For this review, take the finished solid that the model builds, in its own axes (mm). Give positions to 0.01 mm unless a question says otherwise; leave off trailing zeros. Write each loop counter-clockwise with the first axis right and the second up, starting at its lowest first coordinate (ties: lowest second). Pieces come first, ordered by that corner, then holes.
1) We need section B-B on y = 77.5. Give the boundary of the cut face in (x, z).
2) We need section A-A on x = 127. Give the boundary of the cut face in (y, z), and give its area (3 significant figures).
3) We need section C-C on x = 61. Give the boundary of the cut face in (y, z), and give its area (3 significant figures).
4) Wall thickness on line 1 along X through (y, z) = (184.5, 2.3); line 2 along Y through (x, z) = (13, 2.35): over which ranges is each line inside the solid? List them lowest first.
5) We need section D-D on y = 158.5. Give the boundary of the cut face in (x, z), and give its area (3 significant figures).
6) For P1, Ø10, axis at x = 113, y = 106.5, coming from the -Z side; P2, Ø6, axis at x = 174.5, y = 181.5, coming from the +Z side; P3, Ø17, axis at x = 168, y = 105.5, coming from the +Z side, all flat-tipped, find the tip position at first contact; note any pin that passes through.
7) Draft analysis for pull direction Y (two halves, no side actions). For faces 1 (the face through (104, 106, 0)), 2 (the face through (104, 106, 0.8)), 3 (the face through (164, 197, 1.6)), state which applies: pulls with the +Y half, pulls with the -Y half, needs draft (parallel to the pull), parting line crosses it, or undercut.
from build123d import *

# Parameters (mm, degrees)
F0_W     = 210
F0_H     = 210
F1_DEPTH = 0.8
F2_W     = 210
F2_H     = 210
F2_W_2   = 207.12
F2_H_2   = 207.12
F3_DEPTH = 2
F5_DEPTH = 2
F6_W     = 87
F6_H     = 24
F6_W_2   = 21
F6_H_2   = 21
F7_DEPTH = 0.8


with BuildPart() as f1:
    # F0 (on Top) → F1 (new body)
    with BuildSketch(Plane.XY):
        with Locations((105, 105)):
            Rectangle(F0_W, F0_H)
    extrude(amount=F1_DEPTH)

    # F2 (on face) → F3 (join)
    with BuildSketch(Plane.XY.offset(0.8)):
        with Locations((105, 105)):
            Rectangle(F2_W, F2_H)
        with Locations((105, 105)):
            Rectangle(F2_W_2, F2_H_2, mode=Mode.SUBTRACT)
    extrude(amount=F3_DEPTH)

    # F4 (on face) → F5 (join, through all)
    with BuildSketch(Plane.XY.offset(0.8)):
        Polygon((72.889231, 173.372308), (72.889231, 208.56), (71.449231, 208.56), (71.449231, 174.812308), (35.766923, 174.812308), (35.766923, 111.636923), (37.206923, 111.636923), (37.206923, 173.372308), align=None)
    extrude(amount=F5_DEPTH)

    # F6 (on face) → F7 (join)
    with BuildSketch(Plane.XY.offset(0.8)):
        with Locations((165.06, 196.56)):
            Rectangle(F6_W, F6_H)
        with Locations((168.06, 101.06)):
            Rectangle(F6_W_2, F6_H_2)
    extrude(amount=F7_DEPTH)


solid = f1.part
Results list:
1. outline: (0, 0) - (210, 0) - (210, 2.8) - (208.56, 2.8) - (208.56, 0.8) - (1.44, 0.8) - (1.44, 2.8) - (0, 2.8) - close
2. outline: (0, 0) - (210, 0) - (210, 2.8) - (208.56, 2.8) - (208.56, 1.6) - (184.56, 1.6) - (184.56, 0.8) - (1.44, 0.8) - (1.44, 2.8) - (0, 2.8) - close
2. area: 193 mm2
3. outline: (0, 0) - (210, 0) - (210, 2.8) - (208.56, 2.8) - (208.56, 0.8) - (174.81, 0.8) - (174.81, 2.8) - (173.37, 2.8) - (173.37, 0.8) - (1.44, 0.8) - (1.44, 2.8) - (0, 2.8) - close
3. area: 177 mm2
4. line 1: x = 0 to 1.44, 71.45 to 72.89, 208.56 to 210
4. line 2: y = 0 to 1.44, 208.56 to 210
5. outline: (0, 0) - (210, 0) - (210, 2.8) - (208.56, 2.8) - (208.56, 0.8) - (37.21, 0.8) - (37.21, 2.8) - (35.77, 2.8) - (35.77, 0.8) - (1.44, 0.8) - (1.44, 2.8) - (0, 2.8) - close
5. area: 177 mm2
6. P1: stops at z = 0
6. P2: stops at z = 0.8
6. P3: stops at z = 1.6
7. face 1: needs draft
7. face 2: undercut
7. face 3: undercut
